For this review, take the finished solid that the model builds, in its own axes (mm). Coordinates: 2 decimals unless noted, no trailing zeros. Order: outer loops, then holes, each group sorted by start corner. A loop starts at its lowest first (then second) coordinate and runs counter-clockwise, first axis right, second up. Notation, with made-up numbers: (69.5, 16.5) -> (104.5, 16.5) arc R15 cw to (104.5, 38.5) -> close; hole circle Ø3 at (37, -6). An arc over 180 degrees is marked (long way). Return JSON: item names as keys, results as strings. Group by question number.
Item 1: For line 1 along Y through (x, z) = (-1.35, 7); line 2 along Z through (x, y) = (-1.25, -0.75); line 3 along X through (y, z) = (-0.25, -18), list the stretches that pass through material, from the lowest coordinate up.
Item 2: Take a section at A-A (x = 0). Write out the cut boundary in (y, z).
Item 3: Take a section at C-C (z = -81). Write out the cut boundary in (x, y), then the cut area to 3 significant figures.
Item 4: Insertion check: pin 1 (2 mm diameter, centred on x = 4, y = 5.5, fed in from -Z); pin 2 (1.5 mm diameter, centred on y = -5, z = -55.5, fed in from -X); pin 3 (4 mm diameter, centred on y = 0, z = 7, fed in from +X). Each pin has a flat end and moves straight along its axis. Give the tip position at first contact, or say it passes through.
Item 5: Take a section at B-B (y = 0). Write out the cut boundary in (x, z).
Item 6: Take a section at D-D (y = 6). Write out the cut boundary in (x, z).
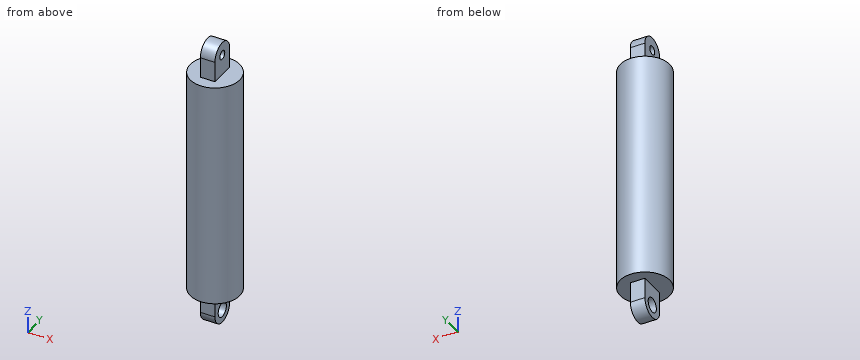
```python
from build123d import *

# Parameters (mm, degrees)
SKETCH1_W           = 78
SKETCH1_H           = 8.5
SKETCH2_R           = 1.5
SKETCH2_R_2         = 2.5
BOSS_EXTRUDE1_DEPTH = 2.5


with BuildPart() as part:
    # Sketch1 → Revolve1 (revolve)
    with BuildSketch(Plane(origin=(0, 0, 0), x_dir=(0, 0, -1), z_dir=(1, 0, 0)), mode=Mode.PRIVATE) as revolve1_sk:
        with Locations((39, 4.25)):
            Rectangle(SKETCH1_W, SKETCH1_H)
    revolve(revolve1_sk.sketch.rotate(Axis((0, 0, 27.669458773), (0, 0, -1)), 90), axis=Axis((0, 0, 27.669458773), (0, 0, -1)))

    # Sketch2 → Boss-Extrude1 (add, symmetric)
    # profile 1 of 2: a face of its own
    with BuildSketch(Plane(origin=(0, 0, 0), x_dir=(0, 0, -1), z_dir=(1, 0, 0))):
        with BuildLine():
            Line((-7, 4.5), (0, 4.5))
            Line((0, 4.5), (0, -4.5))
            Line((0, -4.5), (-7, -4.5))
            ThreePointArc((-7, -4.5), (-11.5, 0), (-7, 4.5))
        make_face()
        with Locations((-7, 0)):
            Circle(SKETCH2_R, mode=Mode.SUBTRACT)
    # profile 2 of 2: a face of its own
    with BuildSketch(Plane(origin=(0, 0, 0), x_dir=(0, 0, -1), z_dir=(1, 0, 0))):
        with BuildLine():
            Line((85, 4.5), (78, 4.5))
            Line((78, 4.5), (78, -4.5))
            Line((78, -4.5), (85, -4.5))
            ThreePointArc((85, -4.5), (89.5, 0), (85, 4.5))
        make_face()
        with Locations((85, 0)):
            Circle(SKETCH2_R_2, mode=Mode.SUBTRACT)
    extrude(amount=BOSS_EXTRUDE1_DEPTH, both=True)


solid = part.part
```
Findings below:
{
 "1": {"line 1": "y = -4.5 to -1.5, 1.5 to 4.5", "line 2": "z = -89.44 to -87.38, -82.62 to 5.7, 8.3 to 11.44", "line 3": "x = -8.5 to 8.5"},
 "2": {"outline": "(-8.5, -78) -> (-4.5, -78) -> (-4.5, -85) arc R4.5 ccw to (4.5, -85) -> (4.5, -78) -> (8.5, -78) -> (8.5, 0) -> (4.5, 0) -> (4.5, 7) arc R4.5 ccw to (-4.5, 7) -> (-4.5, 0) -> (-8.5, 0) -> close; hole circle Ø5 at (0, -85); hole circle Ø3 at (0, 7)"},
 "3": {"outline": "(-2.5, -4.5) -> (2.5, -4.5) -> (2.5, 4.5) -> (-2.5, 4.5) -> close", "area": "45.0 mm2"},
 "4": {"pin 1": "stops at z = -78", "pin 2": "stops at x = -7.36", "pin 3": "stops at x = 2.5"},
 "5": {"outline": "(-8.5, -78) -> (-2.5, -78) -> (-2.5, -82.5) -> (2.5, -82.5) -> (2.5, -78) -> (8.5, -78) -> (8.5, 0) -> (2.5, 0) -> (2.5, 5.5) -> (-2.5, 5.5) -> (-2.5, 0) -> (-8.5, 0) -> close; (-2.5, -89.5) -> (2.5, -89.5) -> (2.5, -87.5) -> (-2.5, -87.5) -> close; (-2.5, 8.5) -> (2.5, 8.5) -> (2.5, 11.5) -> (-2.5, 11.5) -> close"},
 "6": {"outline": "(-6.02, -78) -> (6.02, -78) -> (6.02, 0) -> (-6.02, 0) -> close"}
}
